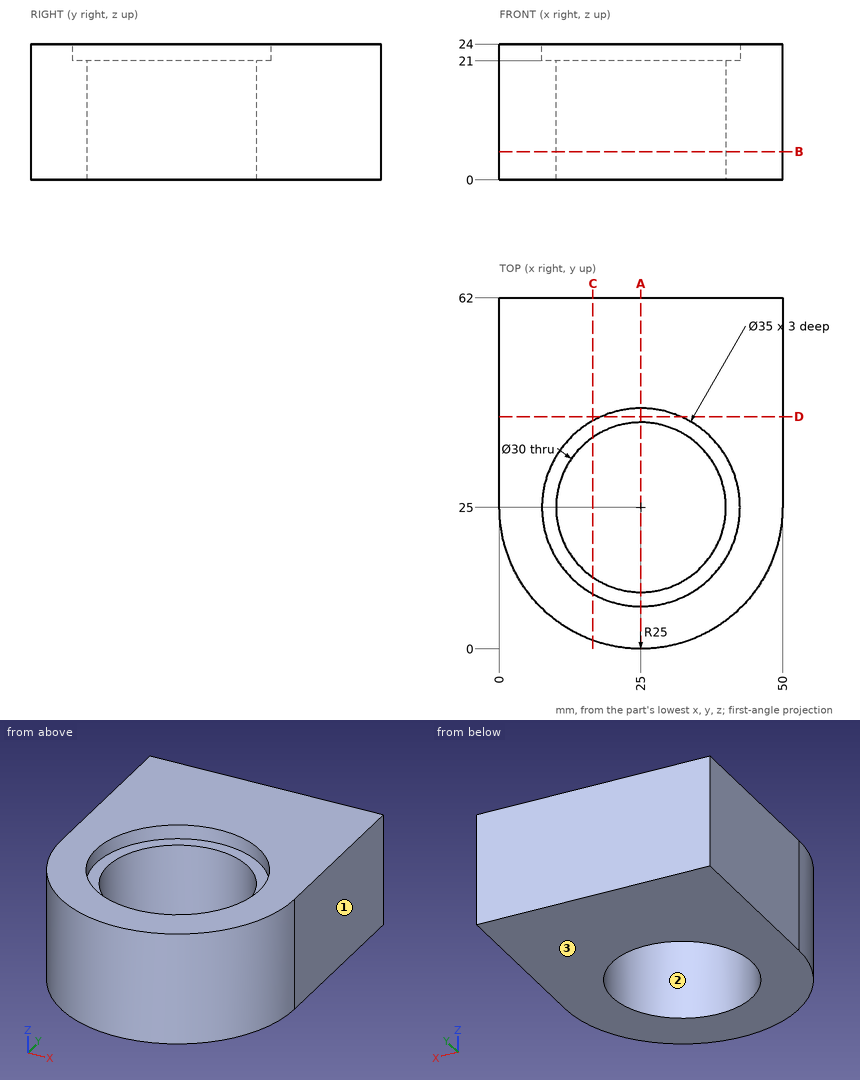
Verification items for this drawing (mm, ordinates from the low corner). Coordinates: 2 decimals unless noted, no trailing zeros. Order: outer loops, then holes, each group sorted by start corner. A loop starts at its lowest first (then second) coordinate and runs counter-clockwise, first axis right, second up.
Q1. Sectioned sample at D-D on y = 41. Record the cut outline in (x, z).
Reply:
outline: (0, 0) - (50, 0) - (50, 24) - (32.09, 24) - (32.09, 21) - (17.91, 21) - (17.91, 24) - (0, 24) - close
Q2. Draft check along X on the marked faces 1, 2 and 3. Enter one of: released by +X, released by -X, zero draft, split by the parting line, or undercut.
Reply:
face 1: released by +X
face 2: undercut
face 3: zero draft
Q3. Depth check by flat-ended pin: pin 1 Ø3 at (x, z) = (9.5, 8.5) entering from -Y; pin 2 Ø1 at (y, z) = (23, 7.5) entering from +X; pin 3 Ø4 at (y, z) = (21.5, 16) entering from -X. Enter the tip coordinate at first touch or a pass-through.
Reply:
pin 1: stops at y = 4.29
pin 2: stops at x = 49.95
pin 3: stops at x = 0.05
Q4. Sectioned sample at A-A on x = 25. Record the cut outline in (y, z).
Reply:
outline: (0, 0) - (10, 0) - (10, 21) - (7.5, 21) - (7.5, 24) - (0, 24) - close; (40, 0) - (62, 0) - (62, 24) - (42.5, 24) - (42.5, 21) - (40, 21) - close
Q5. Sectioned sample at B-B on z = 5. Record the cut outline in (x, y), and give its area (3 significant figures).
Reply:
outline: (0, 25) arc R25 ccw to (50, 25) - (50, 62) - (0, 62) - close; hole circle Ø30 at (25, 25)
area: 2,120 mm2
Q6. Sectioned sample at C-C on x = 16.5. Record the cut outline in (y, z).
Reply:
outline: (1.49, 0) - (12.64, 0) - (12.64, 21) - (9.7, 21) - (9.7, 24) - (1.49, 24) - close; (37.36, 0) - (62, 0) - (62, 24) - (40.3, 24) - (40.3, 21) - (37.36, 21) - close
Q7. Thickness scan on probe 1 along Y at (x, z) = (25, 16.25); probe 2 along Y at (x, z) = (25, 21.95); probe 3 along X at (y, z) = (34.5, 10). Record the ranges inside material, lowest first.
Reply:
probe 1: y = 0 to 10, 40 to 62
probe 2: y = 0 to 7.5, 42.5 to 62
probe 3: x = 0 to 13.39, 36.61 to 50
